Check sheet for the modelled part. Datum: model origin and axes. Units: mm. A direction names the side the tool comes from. Give positions to 0.01 mm unless a question says otherwise; leave off trailing zeros. Loops run counter-clockwise (first coordinate to the right, second up) from the corner with the lowest first, then second, coordinate; pieces in that order, holes last. Notation, with made-up numbers: (28.5, -30) -> (65.5, -30) arc R5 ccw to (65.5, -22) -> close; hole circle Ø5 at (53, 44.25). An arc over 180 degrees is marked (long way). Write each question's results on one line, items separated by ' | '. Start each with the question number.
Item 1: Cross-section at C-C on y = -16. Enter the section's corners in (x, z), then the cut area to 3 significant figures.
Item 2: Mould release check, pull along X, two halves, no side actions. Record for faces 1 (the face through (-1, 30.75, 9)), 2 (the face through (-37.5, 0, 7)), 3 (the face through (-38.25, 0, 9)): pulls with the +X half, pulls with the -X half, needs draft (parallel to the pull), parting line crosses it, or undercut.
Item 3: Cross-section at B-B on z = 13.5. Enter the section's corners in (x, y), then the cut area to 3 significant figures.
Item 4: Scan lines: line 1 along Y through (x, z) = (28, 10); line 2 along X through (y, z) = (8, 8.5); line 3 along Z through (x, y) = (3, 1.5). Record each from-to range of solid material in increasing order.
Item 5: Gauge pin test, flat end, axial feed: pin 1 Ø1 at (x, y) = (28, 2.5) entering from -Z. Record the tip position at first contact, or that the pin passes through.
Item 6: Cross-section at A-A on x = -19. Enter the section's corners in (y, z).
Item 7: Access from +Z, -Z, +X, -X, +Y, -Y to the whole of each face (thin tool, end or side, straight path). Record for faces 4 (the face through (-27.87, 30.38, 11.41)), 5 (the face through (-1, 0, 15)), 6 (the face through (-1, -30.75, 9)).
from build123d import *

# Parameters (mm, degrees)
SKETCH_W        = 76.5
SKETCH_H        = 61.5
PAD_DEPTH       = 18
SKETCH001_W     = 75
SKETCH001_H     = 60
POCKET_DEPTH    = 15
SKETCH003_R     = 3.33
POCKET001_DEPTH = 5


with BuildPart() as part:
    # Sketch → Pad (new body)
    with BuildSketch(Plane.XY):
        Rectangle(SKETCH_W, SKETCH_H)
    extrude(amount=PAD_DEPTH)

    # Sketch001 (on Face5 of Pad) → Pocket (cut)
    with BuildSketch(Plane(origin=(0, 0, 0), x_dir=(1, 0, 0), z_dir=(0, 0, -1))):
        Rectangle(SKETCH001_W, SKETCH001_H)
    extrude(amount=-POCKET_DEPTH, mode=Mode.SUBTRACT)

    # Sketch003 (on Face1 of Pocket) → Pocket001 (cut)
    with BuildSketch(Plane(origin=(0, 30.75, 0), x_dir=(-1, 0, 0), z_dir=(0, 1, 0))):
        with Locations((31.1968, 11.26101)):
            Circle(SKETCH003_R)
    extrude(amount=-POCKET001_DEPTH, mode=Mode.SUBTRACT)


solid = part.part
Answer sheet:
1) outline: (-38.25, 0) -> (-37.5, 0) -> (-37.5, 15) -> (37.5, 15) -> (37.5, 0) -> (38.25, 0) -> (38.25, 18) -> (-38.25, 18) -> close | area: 252 mm²
2) face 1: needs draft | face 2: undercut | face 3: pulls with the -X half
3) outline: (-38.25, -30.75) -> (38.25, -30.75) -> (38.25, 30.75) -> (-28.73, 30.75) -> (-28.73, 30) -> (37.5, 30) -> (37.5, -30) -> (-37.5, -30) -> (-37.5, 30) -> (-33.66, 30) -> (-33.66, 30.75) -> (-38.25, 30.75) -> close | area: 201 mm²
4) line 1: y = -30.75 to -30, 30 to 30.75 | line 2: x = -38.25 to -37.5, 37.5 to 38.25 | line 3: z = 15 to 18
5) pin 1: stops at z = 15
6) outline: (-30.75, 0) -> (-30, 0) -> (-30, 15) -> (30, 15) -> (30, 0) -> (30.75, 0) -> (30.75, 18) -> (-30.75, 18) -> close
7) face 4: +Y | face 5: -Z | face 6: +Z, -Z, +X, -X, -Y
